The listing builds one solid part. Answer for the finished solid, in the listing's coordinates (mm). Give positions to 0.01 mm unless a question says otherwise; leave off trailing zeros. Order: outer loops, then holes, each group sorted by start corner. A loop starts at its lowest first (then second) coordinate and runs counter-clockwise, first axis right, second up. Notation, with made-up numbers: M -39,7.25 L -14,7.25 A10 cw -14,21.25 Z; hole C 79,28.5 d8. An arc over 180 degrees is marked long. Answer as a JSON object with one key per item and string values. Group by question number.
```python
from build123d import *

# Parameters (mm, degrees)
SKETCH1_W              = 101.6
SKETCH1_H              = 71.12
BASE_DEPTH             = 6.35
MOTOR_MOUNTING_HOLES_D = 3.4
SKETCH4_R              = 11
CUT_EXTRUDE1_DEPTH     = 125.181064982


with BuildPart() as part:
    # Sketch1 → base (new body)
    with BuildSketch(Plane.XY):
        with Locations((50.8, 35.56)):
            Rectangle(SKETCH1_W, SKETCH1_H)
    extrude(amount=BASE_DEPTH)

    # motor mounting holes (through all)
    with Locations(Plane.XY.offset(6.35)):
        with Locations((35.3, 46.615), (66.3, 15.615), (35.3, 15.615), (66.3, 46.615)):
            Hole(MOTOR_MOUNTING_HOLES_D / 2)

    # Sketch4 → Cut-Extrude1 (cut, through all)
    with BuildSketch(Plane.XY.offset(6.35)):
        with Locations((50.8, 31.115)):
            Circle(SKETCH4_R)
    extrude(amount=-CUT_EXTRUDE1_DEPTH, mode=Mode.SUBTRACT)


solid = part.part
```
Item 1: Section B-B (y = 22.5) is taken. Determine the outline of the cut face in (x, z).
Item 2: Section C-C (x = 66.3) is taken. Determine the outline of the cut face in (y, z) (3 decimals).
Item 3: Determine the mould class of faces 1 (the cylindrical face through (37, 15.69, 3.13)), 2 (the flat face through (50, 44, 6.35)), 3 (the flat face through (101.6, 35, 3)) for opening direction X: released by +X, released by -X, zero draft, split by the parting line, or undercut.
Item 4: Section A-A (x = 50.8) is taken. Determine the outline of the cut face in (y, z) (3 decimals), and give its area (3 significant figures).
Item 5: Flat-ended cylindrical pins translate along their axes: P1, Ø5.5, axis at x = 35.3, y = 15.615, coming from the +Z side; P2, Ø3, axis at x = 66.3, y = 15.615, coming from the -Z side. Find the tip coordinate at first contact, or state that the pin passes through.
Item 6: Consider probe 1 along Y at (x, z) = (66.3, 2.25) (3 decimals); probe 2 along Y at (x, z) = (50.8, 2.25) (3 decimals); probe 3 along X at (y, z) = (24, 1.75). Determine where each line is inside the solid, lowest interval first. Write a range as from..to.
Values found:
{
 "1": {"outline": "M 0,0 L 43.96,0 L 43.96,6.35 L 0,6.35 Z; M 57.64,0 L 101.6,0 L 101.6,6.35 L 57.64,6.35 Z"},
 "2": {"outline": "M 0,0 L 13.915,0 L 13.915,6.35 L 0,6.35 Z; M 17.315,0 L 44.915,0 L 44.915,6.35 L 17.315,6.35 Z; M 48.315,0 L 71.12,0 L 71.12,6.35 L 48.315,6.35 Z"},
 "3": {"face 1": "undercut", "face 2": "zero draft", "face 3": "released by +X"},
 "4": {"outline": "M 0,0 L 20.115,0 L 20.115,6.35 L 0,6.35 Z; M 42.115,0 L 71.12,0 L 71.12,6.35 L 42.115,6.35 Z", "area": "312 mm^2"},
 "5": {"P1": "stops at z = 6.35", "P2": "passes through"},
 "6": {"probe 1": "y = 0..13.915, 17.315..44.915, 48.315..71.12", "probe 2": "y = 0..20.115, 42.115..71.12", "probe 3": "x = 0..42.41, 59.19..101.6"}
}
